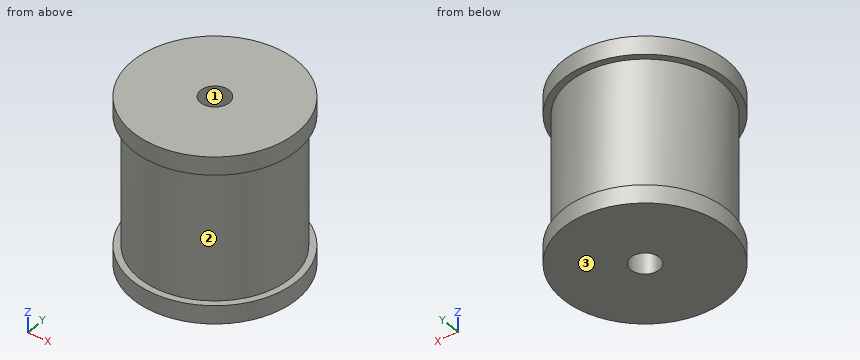
Autodesk Inventor part; units mm, degrees
ref_plane "YZ Plane" through (0, 0, 0) normal (1, 0, 0) x (0, 1, 0)
ref_plane "XZ Plane" through (0, 0, 0) normal (0, 1, 0) x (-1, 0, 0)
ref_plane "XY Plane" through (0, 0, 0) normal (0, 0, 1) x (1, 0, 0)
sketch "Skizze2" plane through (0, 0, 0) normal (0, 1, 0) x (-1, 0, 0)
  line L0 (-5.5, 64) -> (-31.5, 64)
  line L1 (-31.5, 64) -> (-31.5, 57)
  line L2 (-31.5, 57) -> (-29, 57)
  line L3 (-29, 57) -> (-29, 7)
  line L4 (-29, 7) -> (-31.5, 7)
  line L5 (-31.5, 7) -> (-31.5, 0)
  line L6 (-31.5, 0) -> (-5.5, 0)
  line L7 (0, 32) -> (-29, 32) construction
  line L8 (0, 0) -> (0, 64)
  line L9 (-5.5, 64) -> (-5.5, 0)
  point P0 (-5.5, 32)
  dimension "d3" = 7
  dimension "d4" = 64
  dimension "d5" = 11
  dimension "d6" = 63
  dimension "d7" = 58
revolve "Umdrehung1" add sketch "Skizze2" angle 360 about axis through (0, 0, 0) along (0, 0, 1)
properties part number "Kupferspule 500g" material "PC/ABS-Kunststoff"
Can you work these out from the model? Positions are in its coordinate system, mm. Face numbers are marked on the shaded views. Round coordinates to 2 decimals unless told otherwise and drop trailing zeros. Loops run counter-clockwise (first coordinate to the right, second up) from the corner with the lowest first, then second, coordinate; pieces in that order, holes last. Notation, with made-up numbers: (-38.75, 7) - (-23.75, 7) arc R14 ccw to (-23.75, 13) - close; hole circle Ø7 at (88.25, 77). An arc over 180 degrees is marked (long way). Answer in a Markdown table with one row per item. Add a question column.
Q1. I want a section at D-D on y = 25. List the corners of the cut face in (x, z) for me, and give its area (3 significant figures).
Q2. I want a section at A-A on y = 0. List the corners of the cut face in (x, z) for me, and give its area (3 significant figures).
Q3. We'd pull the mould along Y, two halves only. Please class the marked faces 1, 2 and 3: pulls with the +Y half, pulls with the -Y half, needs draft (parallel to the pull), parting line crosses it, or undercut.
Q4. I want a section at C-C on z = 9. List the corners of the cut face in (x, y) for me.
Q5. I need wall thicknesses on L1, parallel to Y at x = 0, z = 42.5; L2, parallel to Z at x = 26, y = 15.5; L3, parallel to Y at x = 1, z = 16.5. Which ranges of each line are inside material? Lowest first, please.
Q6. For pin 1 Ø10 at (y, z) = (-14.5, 30) entering from -X; pin 2 Ø10 at (y, z) = (-22, 56.5) entering from +X; pin 3 Ø3 at (x, z) = (-7, 29) entering from +Y, each with a flat end and sliding along its axis, tell me the tip position at first contact or that it passes through.
A:
| question | item | result |
|---|---|---|
| 1 | outline | (-19.16, 0) - (19.16, 0) - (19.16, 7) - (14.7, 7) - (14.7, 57) - (19.16, 57) - (19.16, 64) - (-19.16, 64) - (-19.16, 57) - (-14.7, 57) - (-14.7, 7) - (-19.16, 7) - close |
| 1 | area | 2,010 mm^2 |
| 2 | outline | (-31.5, 0) - (-5.5, 0) - (-5.5, 64) - (-31.5, 64) - (-31.5, 57) - (-29, 57) - (-29, 7) - (-31.5, 7) - close; (5.5, 0) - (31.5, 0) - (31.5, 7) - (29, 7) - (29, 57) - (31.5, 57) - (31.5, 64) - (5.5, 64) - close |
| 2 | area | 3,080 mm^2 |
| 3 | face 1 | undercut |
| 3 | face 2 | parting line crosses it |
| 3 | face 3 | needs draft |
| 4 | outline | circle Ø58 at (0, 0); hole circle Ø11 at (0, 0) |
| 5 | L1 | -29 to -5.5, 5.5 to 29 |
| 5 | L2 | 0 to 7, 57 to 64 |
| 5 | L3 | -28.98 to -5.41, 5.41 to 28.98 |
| 6 | pin 1 | x = -27.4 |
| 6 | pin 2 | x = 26.5 |
| 6 | pin 3 | y = 28.47 |
